CAD build for the part. Positions are in the model's coordinates, mm. Round coordinates to 2 decimals unless told otherwise and drop trailing zeros. Write each loop counter-clockwise with the first axis right and the second up, starting at its lowest first coordinate (ties: lowest second). Pieces come first, ordered by that corner, then holes. Notation, with made-up numbers: (-6.75, 7.5) - (-0.75, 7.5) arc R22 cw to (-0.75, 42.5) - close; hole circle Ø5 at (40.25, 60). An arc over 180 degrees is marked (long way). Put each result on its own line as item: value. Start each with the question number.
Item 1: Cut at B-B (z = 69.5). Give the cut face in (x, y), and give its area (3 significant figures).
Item 2: Cut at A-A (x = -350). Give the cut face in (y, z).
Item 3: Cut at D-D (y = 87). Give the cut face in (x, z), and give its area (3 significant figures).
Item 4: Cut at C-C (z = 118.5). Give the cut face in (x, y).
Item 5: Drill centre lines: line 1 (Y direction, x = -213, z = 51); line 2 (X direction, y = 334, z = 99.5); line 3 (X direction, y = 199.5, z = 180). Where is each one in solid material? Low to high. Write a range as from..to.
```python
from build123d import *

# Parameters (mm, degrees)
SKETCH3_W           = 400
SKETCH3_H           = 300
BOSS_EXTRUDE2_DEPTH = 1050
FILLET1_R           = 110
CHAMFER1_SIZE       = 200
CHAMFER1_SIZE2      = 93.261531631
SKETCH4_R           = 15
BOSS_EXTRUDE3_DEPTH = 50


with BuildPart() as part:
    # Sketch3 → Boss-Extrude2 (new body)
    with BuildSketch(Plane(origin=(0, 0, 0), x_dir=(0, 0, -1), z_dir=(1, 0, 0))):
        with Locations((0, 200)):
            Rectangle(SKETCH3_W, SKETCH3_H)
    extrude(amount=-BOSS_EXTRUDE2_DEPTH)

    # Fillet1
    fillet1_edges = [part.edges().sort_by_distance(p)[0] for p in [
        (0, 350, 0),
        (0, 200, -200),
        (0, 50, 0),
        (0, 200, 200),
    ]]
    fillet(fillet1_edges, radius=FILLET1_R)

    # Chamfer1
    chamfer1_edges = [part.edges().sort_by_distance(p)[0] for p in [
        (-1050, 350, 0),
    ]]
    chamfer1_side = [part.faces().sort_by_distance(p)[0] for p in [
        (-580, 350, 0),
    ]]
    chamfer(chamfer1_edges, length=CHAMFER1_SIZE, length2=CHAMFER1_SIZE2, reference=chamfer1_side[0])

    # Sketch4 → Boss-Extrude3 (add)
    with BuildSketch(Plane.XZ.offset(-50)):
        with Locations(Location((-850, 165, 0), (0, 0, 270))):
            Circle(SKETCH4_R)
        with Locations(Location((-350, 165, 0), (0, 0, 270))):
            Circle(SKETCH4_R)
        with Locations(Location((-350, -165, 0), (0, 0, 90))):
            Circle(SKETCH4_R)
        with Locations(Location((-850, -165, 0), (0, 0, 90))):
            Circle(SKETCH4_R)
    extrude(amount=BOSS_EXTRUDE3_DEPTH)


solid = part.part
```
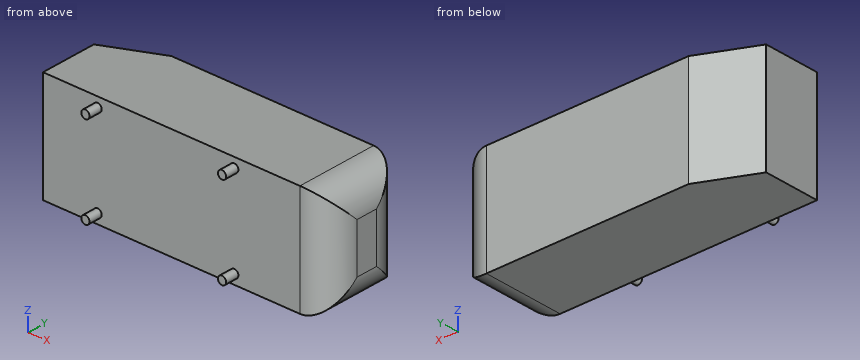
Output values:
1. outline: (-1050, 50) - (-110, 50) arc R110 ccw to (0, 160) - (0, 240) arc R110 ccw to (-110, 350) - (-850, 350) - (-1050, 256.74) - close
1. area: 300,000 mm2
2. outline: (0, -180) - (50, -180) - (50, -200) - (350, -200) - (350, 200) - (50, 200) - (50, 180) - (0, 180) - (0, 150) - (50, 150) - (50, -150) - (0, -150) - close
3. outline: (-1050, -200) - (-110, -200) arc R110 ccw to (-27.71, -163) - (-27.71, 163) arc R110 ccw to (-110, 200) - (-1050, 200) - close
3. area: 407,000 mm2
4. outline: (-1050, 50) - (-110, 50) arc R110 ccw to (-3.76, 131.5) - (-3.76, 268.5) arc R110 ccw to (-110, 350) - (-850, 350) - (-1050, 256.74) - close
5. line 1: 50..350
5. line 2: -884.31..-52.87
5. line 3: -1050..-46.75
